Source: CAD feature listing. Evaluate the final solid. Frame: model axes, mm. A direction names the side the tool comes from. Give positions to 0.01 mm unless a question says otherwise; leave off trailing zeros. Order: outer loops, then holes, each group sorted by start corner. A loop starts at its lowest first (then second) coordinate and runs counter-clockwise, first axis right, second up.
```python
from build123d import *

# Parameters (mm, degrees)
F0_R     = 2.6035
F1_DEPTH = 25.4


# Not quite as in the source:
# - ends of sketch curves that miss each other by under 0.0002 mm in the source are joined


with BuildPart() as f1:
    # F0 (on Front) → F1 (new body)
    with BuildSketch(Plane.XZ):
        with BuildLine():
            ThreePointArc((-12.6999998568, 10.5791116031), (-12.1919492, 10.06475), (-12.6999998568, 9.5503883969))
            Line((-12.6999998568, 9.5503883969), (-12.7, 6.35))
            ThreePointArc((-12.7, 6.35), (-12.4953913266, 3.565448735), (-11.8859605514, 0.8407130437))
            ThreePointArc((-11.8859605514, 0.8407130437), (-11.2503853868, 0.5162584682), (-11.5663491172, -0.1235908641))
            ThreePointArc((-11.5663491172, -0.1235908641), (-11.0492007439, -1.4069525893), (-10.4402782322, -2.6493920286))
            ThreePointArc((-10.4402782322, -2.6493920286), (-9.7531608674, -2.84205605), (-9.9366469283, -3.5316852695))
            ThreePointArc((-9.9366469283, -3.5316852695), (-7.1203841816, -7.1203841816), (-3.5316659689, -9.9366564303))
            ThreePointArc((-3.5316659689, -9.9366564303), (-2.84205605, -9.7531608674), (-2.6494036278, -10.4402857754))
            ThreePointArc((-2.6494036278, -10.4402857754), (-1.4069525893, -11.0492007439), (-0.1235924101, -11.5663361575))
            ThreePointArc((-0.1235924101, -11.5663361575), (0.5162584682, -11.2503853868), (0.8407328825, -11.8859611899))
            ThreePointArc((0.8407328825, -11.8859611899), (3.565448735, -12.4953913266), (6.35, -12.7))
            Line((6.35, -12.7), (9.5504, -12.7))
            ThreePointArc((9.5504, -12.7), (10.06475, -12.1919492), (10.5791116031, -12.6999998568))
            ThreePointArc((10.5791116031, -12.6999998568), (12.0825733161, -12.0825733161), (12.7000122396, -10.579099926))
            ThreePointArc((12.7000122396, -10.579099926), (12.1919492, -10.06475), (12.6999998568, -9.5503883969))
            Line((12.6999998568, -9.5503883969), (12.7, -6.3246))
            ThreePointArc((12.7, -6.3246), (12.192, -5.8166), (12.7, -5.3086))
            Line((12.7, -5.3086), (12.7, -4.3023028))
            ThreePointArc((12.7, -4.3023028), (11.5951, -3.1974028), (10.4902, -4.3023028))
            Line((10.4902, -4.3023028), (10.4902, -6.4747902))
            ThreePointArc((10.4902, -6.4747902), (9.8630063673, -7.413451805), (8.7557795103, -7.1932106897))
            Line((8.7557795103, -7.1932106897), (5.4384448, -3.8758622))
            ThreePointArc((5.4384448, -3.8758622), (4.7501824843, -2.8458268978), (4.5085, -1.630807))
            Line((4.5085, -1.630807), (4.5085, 1.630807))
            ThreePointArc((4.5085, 1.630807), (4.7501824843, 2.8458268978), (5.4384359697, 3.8758710303))
            Line((5.4384359697, 3.8758710303), (8.7557864, 7.1932038))
            ThreePointArc((8.7557864, 7.1932038), (9.8630063673, 7.413451805), (10.4902, 6.4747902))
            Line((10.4902, 6.4747902), (10.4902, 4.3023028))
            ThreePointArc((10.4902, 4.3023028), (11.5951, 3.1974028), (12.7, 4.3023028))
            Line((12.7, 4.3023028), (12.7, 5.3086))
            ThreePointArc((12.7, 5.3086), (12.192, 5.8166), (12.7, 6.3246))
            Line((12.7, 6.3246), (12.7, 9.5504))
            ThreePointArc((12.7, 9.5504), (12.1919492, 10.06475), (12.6999998568, 10.5791116031))
            ThreePointArc((12.6999998568, 10.5791116031), (12.0825733161, 12.0825733161), (10.579099926, 12.7000122396))
            ThreePointArc((10.579099926, 12.7000122396), (10.06475, 12.1919492), (9.5503883969, 12.6999998568))
            Line((9.5503883969, 12.6999998568), (6.3246, 12.7))
            ThreePointArc((6.3246, 12.7), (5.8166, 12.192), (5.3086, 12.7))
            Line((5.3086, 12.7), (4.3023028, 12.7))
            ThreePointArc((4.3023028, 12.7), (3.1974028, 11.5951), (4.3023028, 10.4902))
            Line((4.3023028, 10.4902), (6.4747902, 10.4902))
            ThreePointArc((6.4747902, 10.4902), (7.413451805, 9.8630063673), (7.1932106897, 8.7557795103))
            Line((7.1932106897, 8.7557795103), (3.8758622, 5.4384448))
            ThreePointArc((3.8758622, 5.4384448), (2.8458268978, 4.7501824843), (1.630807, 4.5085))
            Line((1.630807, 4.5085), (-1.630807, 4.5085))
            ThreePointArc((-1.630807, 4.5085), (-2.8458268978, 4.7501824843), (-3.8758710303, 5.4384359697))
            Line((-3.8758710303, 5.4384359697), (-7.1932038, 8.7557864))
            ThreePointArc((-7.1932038, 8.7557864), (-7.413451805, 9.8630063673), (-6.4747902, 10.4902))
            Line((-6.4747902, 10.4902), (-4.3023028, 10.4902))
            ThreePointArc((-4.3023028, 10.4902), (-3.1974028, 11.5951), (-4.3023028, 12.7))
            Line((-4.3023028, 12.7), (-5.3086, 12.7))
            ThreePointArc((-5.3086, 12.7), (-5.8166, 12.192), (-6.3246, 12.7))
            Line((-6.3246, 12.7), (-9.5504, 12.7))
            ThreePointArc((-9.5504, 12.7), (-10.06475, 12.1919492), (-10.5791116031, 12.6999998568))
            ThreePointArc((-10.5791116031, 12.6999998568), (-12.0825733161, 12.0825733161), (-12.6999998568, 10.5791116031))
        make_face()
        with BuildLine():
            ThreePointArc((-10.4896860957, 6.4822831536), (-9.8588365186, 7.4144880425), (-8.7552969103, 7.1927280897))
            Line((-8.7552969103, 7.1927280897), (-5.3427122, 3.7801296))
            ThreePointArc((-5.3427122, 3.7801296), (-4.5640049581, 2.5033128493), (-4.4562086701, 1.0116578151))
            ThreePointArc((-4.4562086701, 1.0116578151), (-3.1300157893, -3.1300157893), (1.0116576108, -4.4562074473))
            ThreePointArc((1.0116576108, -4.4562074473), (2.5033128493, -4.5640049581), (3.7801384303, -5.3427033697))
            Line((3.7801384303, -5.3427033697), (7.1927212, -8.7553038))
            ThreePointArc((7.1927212, -8.7553038), (7.4144880425, -9.8588365186), (6.4822831536, -10.4896860957))
            ThreePointArc((6.4822831536, -10.4896860957), (-5.5578196165, -5.5578196165), (-10.4896860957, 6.4822831536))
        make_face(mode=Mode.SUBTRACT)
        Circle(F0_R, mode=Mode.SUBTRACT)
    extrude(amount=F1_DEPTH)


solid = f1.part
```
1) Material intervals for L1, parallel to Z at x = 9.5, y = -6; L2, parallel to Z at x = 0, y = -6.75; L3, parallel to Z at x = -2.25, y = -7.5, sorted ascending.
Report:
L1: z = -12.7 to -7.49, 7.49 to 12.7
L2: z = -11.37 to -9.25, -4.52 to -2.6, 2.6 to 4.51
L3: z = -10.65 to -8.13, -3.82 to -1.31, 1.31 to 4.57
2) Section query C-C, the plane y = -3.5. Count the separate pieces of the cut face and the enclosed holes in it, and give its area (3 significant figures).
Report:
separate pieces: 1
enclosed holes: 2
area: 269 mm2
3) Reachability of faces 5 (the cylindrical face through (10.076, -12.522, 12.192)), 6 (the cylindrical face through (2.483, -12.522, -4.558)) from +Z, -Z, +X, -X, +Y, -Y: full face, straight path, thin tool, end or side. Return the list, or none.
Report:
face 5: +Z, +Y, -Y
face 6: +Y, -Y
4) Section query B-B, the plane x = 2. Return the cut outline in (y, z).
Report:
outline: (-25.4, -12.2) - (0, -12.2) - (0, -9.92) - (-25.4, -9.92) - close; (-25.4, -4.45) - (0, -4.45) - (0, -1.67) - (-25.4, -1.67) - close; (-25.4, 1.67) - (0, 1.67) - (0, 4.53) - (-25.4, 4.53) - close
5) Pin query (flat end, axial travel): pin 1 (1.7 mm diameter, centred on x = -5, y = -9, fed in from -Z); pin 2 (1 mm diameter, centred on x = 1.5, y = -4.5, fed in from +Z); pin 3 (3.5 mm diameter, centred on y = -6.5, z = 0, fed in from +X). Return the tip coordinate at first contact, or that it passes through.
Report:
pin 1: stops at z = -9.55
pin 2: stops at z = 4.53
pin 3: stops at x = 4.51
6) Section query D-D, the plane x = -0.75. Return the cut outline in (y, z).
Report:
outline: (-25.4, -11.33) - (0, -11.33) - (0, -8.92) - (-25.4, -8.92) - close; (-25.4, -4.42) - (0, -4.42) - (0, -2.49) - (-25.4, -2.49) - close; (-25.4, 2.49) - (0, 2.49) - (0, 4.51) - (-25.4, 4.51) - close
7) Section query A-A, the plane x = 8.25. Return the cut outline in (y, z), and give its area (3 significant figures).
Report:
outline: (-25.4, -12.7) - (0, -12.7) - (0, -6.69) - (-25.4, -6.69) - close; (-25.4, 6.69) - (0, 6.69) - (0, 12.7) - (-25.4, 12.7) - close
area: 305 mm2
8) Draft query along Z for faces 1 (the cylindrical face through (-5.805, -12.522, 12.192)), 2 (the cylindrical face through (12.192, -12.522, 10.054)), 3 (the cylindrical face through (2.483, -12.522, 0.782)), 4 (the flat face through (3, -25.4, 0)). Return one class per face: +Z half, -Z half, draft (parallel to the pull), parting line (faces both ways), or undercut.
Report:
face 1: +Z half
face 2: undercut
face 3: undercut
face 4: draft
